Autodesk Inventor part; units mm, degrees
ref_plane "YZ Plane" through (0, 0, 0) normal (1, 0, 0) x (0, 1, 0)
ref_plane "XZ Plane" through (0, 0, 0) normal (0, 1, 0) x (-1, 0, 0)
ref_plane "XY Plane" through (0, 0, 0) normal (0, 0, 1) x (1, 0, 0)
sketch "Sketch1" plane through (0, 0, 0) normal (0, 1, 0) x (-1, 0, 0)
  circle A0 centre (52.8488, -66.0197) radius 22.5
  arc A1 (55.8488, -77.6386) -> (49.8488, -77.6386) centre (52.8488, -66.0197) ccw
  line L0 (52.8488, -88.5197) -> (52.8488, -133.5197)
  line L1 (52.8488, -88.5197) -> (97.8488, -88.5197) construction
  line L2 (52.8488, -133.5197) -> (52.8488, -149.5197)
  circle A2 centre (52.8488, -133.5197) radius 9
  line L3 (52.8488, -133.5197) -> (68.8488, -133.5197)
  line L4 (52.8488, -133.5197) -> (60.8488, -147.3761)
  line L5 (52.8488, -133.5197) -> (68.8488, -133.5197) construction
  line L6 (52.8488, -133.5197) -> (44.8488, -147.3761)
  line L7 (52.8488, -133.5197) -> (68.8488, -133.5197) construction
  line L8 (52.8488, -133.5197) -> (49.8488, -133.5197)
  arc A3 (36.8488, -133.5197) -> (68.8488, -133.5197) centre (52.8488, -133.5197) ccw
  line L9 (52.8488, -66.0197) -> (75.3488, -66.0197)
  line L10 (52.8488, -66.0197) -> (30.3488, -66.0197)
  line L11 (75.3488, -66.0197) -> (68.8488, -133.5197)
  line L12 (30.3488, -66.0197) -> (36.8488, -133.5197)
  line L13 (52.8488, -78.0197) -> (55.8488, -78.0197)
  line L14 (52.8488, -78.0197) -> (55.8488, -78.0197) construction
  line L15 (55.8488, -78.0197) -> (55.8488, -86.0197)
  line L16 (55.8488, -86.0197) -> (49.8488, -86.0197)
  line L17 (52.8488, -78.0197) -> (49.8488, -78.0197)
  line L18 (52.8488, -78.0197) -> (55.8488, -78.0197) construction
  line L19 (49.8488, -78.0197) -> (49.8488, -86.0197)
  line L20 (55.8488, -78.0197) -> (55.8488, -77.6386)
  line L21 (49.8488, -78.0197) -> (49.8488, -77.6386)
  point P0 (0, 0)
  point P1 (30.7622, -70.3132)
  point P2 (74.9353, -70.3132)
  dimension "d0" = 45
  dimension "d1" = 24
  dimension "d2" = 45
  dimension "d3" = 90
  dimension "d4" = 18
  dimension "d5" = 16
  dimension "d6" = 16
  dimension "d7" = 60
  dimension "d8" = 16
  dimension "d9" = 120
  dimension "d10" = 16
  dimension "d11" = 16
  dimension "d12" = 3
  dimension "d13" = 0
  dimension "d14" = 8
  dimension "d15" = 6
  dimension "d16" = 3
  dimension "d17" = 180
extrude "Extrusion1" add sketch "Sketch1" along normal blind 32 contours L9 A1 L10 A0 | L11 A0 L12 L10 A1 L21 L19 L16 L15 L20 L9
extrude "Extrusion2" add sketch "Sketch1" along normal blind 16 contours L11 L3 A2 L0 A0 | A0 L0 A2 L6 A3 L12 | A3 L4 A2 L3 | A3 L2 A2 L4 | L6 A2 L2 A3
properties part number "trial 3"
Could you check a few things on this model? Use its own coordinates, in mm. A direction names the side the tool comes from. Coordinates: 2 decimals unless noted, no trailing zeros. Loops run counter-clockwise (first coordinate to the right, second up) from the corner with the lowest first, then second, coordinate; pieces in that order, holes last.
1. Imagine slicing it at A-A (y = 14.5). Please give me the cut outline in (x, z), and give its area (3 significant figures).
2. Imagine slicing it at C-C (x = -48). Please give me the cut outline in (y, z), and give its area (3 significant figures).
3. Imagine slicing it at D-D (y = 20). Please give me the cut outline in (x, z).
4. For faces 1 (the face through (-33.553, 8.665, -99.297)), 2 (the face through (-53.283, 23.888, -88.516)), 3 (the face through (-49.849, 16, -82)), which set-ups out of +Z, -Z, +X, -X, +Y, -Y let a thin tool reach every point of the face, with its end or its side?
5. We'd pull the mould along Z, two halves only. Please class faces 4 (the face through (-50.898, 7.888, -124.734)), 5 (the face through (-72.144, 8.665, -99.297)), 6 (the face through (-63, 32, -76)): released by +Z, released by -Z, zero draft, split by the parting line, or undercut.
6. For P1, Ø3, axis at x = -53.5, y = 18, coming from the +Z side; P2, Ø10, axis at y = 13.5, z = -90, coming from the +X side; P3, Ø1, axis at x = -69.5, y = 19, coming from the +Z side, each with a flat end and sliding along its axis, tell me the tip position at first contact or that it passes through.
7. I need wall thicknesses on L1, parallel to Z at x = -58, y = 5; L2, parallel to Z at x = -49, y = 5; L3, parallel to Y at x = -39.5, z = -132. Which ranges of each line are inside material? Lowest first, please.
8. Imagine slicing it at B-B (z = -125.5). Please give me the cut outline in (x, y).
Computed values:
1. outline: (-75.35, -66.02) - (-68.85, -133.52) arc R16 ccw to (-36.85, -133.52) - (-30.35, -66.02) arc R22.5 ccw to start; hole circle Ø18 at (-52.85, -133.52); hole (-55.85, -86.02) - (-49.85, -86.02) - (-49.85, -77.64) arc R12 ccw (long way) to (-55.85, -77.64) - close
1. area: 3,040 mm2
2. outline: (0, -148.77) - (16, -148.77) - (16, -141.1) - (0, -141.1) - close; (0, -125.94) - (16, -125.94) - (16, -87.99) - (32, -87.99) - (32, -77) - (0, -77) - close; (0, -55.04) - (32, -55.04) - (32, -44.05) - (0, -44.05) - close
2. area: 1,430 mm2
3. outline: (-75.35, -66.02) - (-74.94, -70.31) arc R22.5 ccw to (-30.76, -70.31) - (-30.35, -66.02) arc R22.5 ccw to start; hole (-55.85, -86.02) - (-49.85, -86.02) - (-49.85, -77.64) arc R12 ccw (long way) to (-55.85, -77.64) - close
4. face 1: -Z, +X, +Y, -Y
4. face 2: -Z, +Y
4. face 3: +Y, -Y
5. face 4: undercut
5. face 5: released by -Z
5. face 6: zero draft
6. P1: stops at z = -43.52
6. P2: stops at x = -32.18
6. P3: stops at z = -50.35
7. L1: z = -148.67 to -140.9, -126.14 to -76.86, -55.18 to -44.12
7. L2: z = -149.05 to -141.66, -125.38 to -77.39, -54.65 to -43.85
7. L3: y = 0 to 16
8. outline: (-69.62, 0) - (-56.93, 0) - (-56.93, 16) - (-69.62, 16) - close; (-48.76, 0) - (-36.08, 0) - (-36.08, 16) - (-48.76, 16) - close
